Source: CAD feature listing. Evaluate the final solid. Frame: model axes, mm. Face numbers are marked on the shaded views. Give positions to 0.01 mm unless a question says otherwise; leave off trailing zeros. Loops run counter-clockwise (first coordinate to the right, second up) from the corner with the lowest first, then second, coordinate; pieces in that order, holes last.
from build123d import *

# Parameters (mm, degrees)
BOSS_EXTRUDE1_DEPTH = 10
BOSS_EXTRUDE2_START = -3
SKETCH2_R           = 3.5
SKETCH2_R_2         = 7.5
BOSS_EXTRUDE2_DEPTH = 3
BOSS_EXTRUDE5_START = -3
BOSS_EXTRUDE5_DEPTH = 10
SKETCH6_R           = 8.5
CUT_EXTRUDE1_DEPTH  = 246.440929757
SKETCH7_R           = 1
CUT_EXTRUDE2_DEPTH  = 246.544802429
BOSS_EXTRUDE6_DEPTH = 22
BOSS_EXTRUDE7_DEPTH = 2
FILLET1_R           = 2
FILLET3_R           = 2
SKETCH11_W          = 12
SKETCH11_H          = 7
CUT_EXTRUDE3_DEPTH  = 247.512170095
BOSS_EXTRUDE8_START = -10
BOSS_EXTRUDE8_DEPTH = 29.65
SKETCH13_R          = 2.5
CUT_EXTRUDE4_DEPTH  = 250.845097028
SKETCH14_W          = 120
SKETCH14_H          = 65
SKETCH14_R          = 5
BOSS_EXTRUDE9_DEPTH = 29.65
SKETCH15_W          = 60
SKETCH15_H          = 55
CUT_EXTRUDE5_DEPTH  = 19.65


with BuildPart() as part:
    # Sketch1 → Boss-Extrude1 (new body)
    with BuildSketch(Plane(origin=(0, 0, 0), x_dir=(1, 0, 0), z_dir=(0, 1, 0))):
        with BuildLine():
            Line((30, 26.5), (30, -243.5))
            Line((30, -243.5), (-30, -243.5))
            Line((-30, -243.5), (-30, 26.5))
            ThreePointArc((-30, 26.5), (0, 56.5), (30, 26.5))
        make_face()
        with BuildLine():
            ThreePointArc((11.477382224, -17.586065429), (21, 0), (11.477382224, 17.586065429))
            Line((11.477382224, 17.586065429), (5.68518373, 33.5))
            Line((5.68518373, 33.5), (-5.68518373, 33.5))
            Line((-5.68518373, 33.5), (-11.477382224, 17.586065429))
            ThreePointArc((-11.477382224, 17.586065429), (-21, 0), (-11.477382224, -17.586065429))
            Line((-11.477382224, -17.586065429), (-5.68518373, -33.5))
            Line((-5.68518373, -33.5), (5.68518373, -33.5))
            Line((5.68518373, -33.5), (11.477382224, -17.586065429))
        make_face(mode=Mode.SUBTRACT)
    extrude(amount=BOSS_EXTRUDE1_DEPTH)

    # Sketch2 → Boss-Extrude2 (add)
    with BuildSketch(Plane(origin=(0, 10, 0), x_dir=(1, 0, 0), z_dir=(0, 1, 0)).offset(BOSS_EXTRUDE2_START)):
        with BuildLine():
            Line((5.68518373, 33.5), (11.477382224, 17.586065429))
            ThreePointArc((11.477382224, 17.586065429), (21, 0), (11.477382224, -17.586065429))
            Line((11.477382224, -17.586065429), (5.68518373, -33.5))
            Line((5.68518373, -33.5), (-5.68518373, -33.5))
            Line((-5.68518373, -33.5), (-11.477382224, -17.586065429))
            ThreePointArc((-11.477382224, -17.586065429), (-21, 0), (-11.477382224, 17.586065429))
            Line((-11.477382224, 17.586065429), (-5.68518373, 33.5))
            Line((-5.68518373, 33.5), (5.68518373, 33.5))
        make_face()
        with Locations(Location((0, 26.5, 0), (0, 0, 270))):
            Circle(SKETCH2_R, mode=Mode.SUBTRACT)
        with Locations(Location((0, -26.5, 0), (0, 0, 90))):
            Circle(SKETCH2_R, mode=Mode.SUBTRACT)
        with Locations(Location((0, 0, 0), (0, 0, 270))):
            Circle(SKETCH2_R_2, mode=Mode.SUBTRACT)
    extrude(amount=BOSS_EXTRUDE2_DEPTH)

    # Sketch5 → Boss-Extrude5 (add)
    with BuildSketch(Plane.XZ.offset(-7).offset(BOSS_EXTRUDE5_START)):
        with BuildLine():
            Line((11.477382224, -17.586065429), (5.68518373, -33.5))
            Line((5.68518373, -33.5), (-5.68518373, -33.5))
            Line((-5.68518373, -33.5), (-11.477382224, -17.586065429))
            ThreePointArc((-11.477382224, -17.586065429), (0, -21), (11.477382224, -17.586065429))
        make_face()
        with BuildLine():
            Line((5.68518373, 33.5), (11.477382224, 17.586065429))
            ThreePointArc((11.477382224, 17.586065429), (0, 21), (-11.477382224, 17.586065429))
            Line((-11.477382224, 17.586065429), (-5.68518373, 33.5))
            Line((-5.68518373, 33.5), (5.68518373, 33.5))
        make_face()
    extrude(amount=BOSS_EXTRUDE5_DEPTH)

    # Sketch6 → Cut-Extrude1 (cut, through all)
    with BuildSketch(Plane.XZ.offset(-7)):
        with Locations(Location((0, 0, 0), (0, 0, 270))):
            Circle(SKETCH6_R)
    extrude(amount=-CUT_EXTRUDE1_DEPTH, mode=Mode.SUBTRACT)

    # Sketch7 → Cut-Extrude2 (cut, through all)
    with BuildSketch(Plane.XZ):
        with Locations(Location((0, 129.5, 0), (0, 0, 270))):
            Circle(SKETCH7_R)
        with Locations(Location((0, 177.5, 0), (0, 0, 90))):
            Circle(SKETCH7_R)
        with BuildLine():
            Line((-12.002194303, 178.230116364), (-24.730116364, 165.502194303))
            Line((-24.730116364, 165.502194303), (-19.780368896, 160.552446834))
            ThreePointArc((-19.780368896, 160.552446834), (14.849242405, 138.650757595), (-7.052446834, 173.280368896))
            Line((-7.052446834, 173.280368896), (-12.002194303, 178.230116364))
        make_face()
    extrude(amount=-CUT_EXTRUDE2_DEPTH, mode=Mode.SUBTRACT)

    # Sketch9 → Boss-Extrude6 (add)
    with BuildSketch(Plane.XZ):
        with BuildLine():
            Line((-21.664213552, 161.224108438), (-19.780368896, 160.552446834))
            ThreePointArc((-19.780368896, 160.552446834), (14.849242405, 138.650757595), (-7.052446834, 173.280368896))
            Line((-7.052446834, 173.280368896), (-7.724108438, 175.164213552))
            ThreePointArc((-7.724108438, 175.164213552), (16.263455967, 137.236544033), (-21.664213552, 161.224108438))
        make_face()
    extrude(amount=-BOSS_EXTRUDE6_DEPTH)

    # Sketch10 → Boss-Extrude7 (add)
    with BuildSketch(Plane(origin=(0, 22, 0), x_dir=(1, 0, 0), z_dir=(0, 1, 0))):
        with BuildLine():
            Line((-21.664213552, -161.224108438), (-16.012679582, -159.209123628))
            ThreePointArc((-16.012679582, -159.209123628), (12.02081528, -141.47918472), (-5.709123628, -169.512679582))
            Line((-5.709123628, -169.512679582), (-7.724108438, -175.164213552))
            ThreePointArc((-7.724108438, -175.164213552), (16.263455967, -137.236544033), (-21.664213552, -161.224108438))
        make_face()
    extrude(amount=BOSS_EXTRUDE7_DEPTH)

    # Fillet1
    fillet1_edges = [part.edges().sort_by_distance(p)[0] for p in [
        (16.263455967, 24, 137.236544033),
    ]]
    fillet(fillet1_edges, radius=FILLET1_R)

    # Fillet3
    # the kernel refuses this fillet: 2 mm, written as the material it adds along each edge
    with BuildSketch(Plane(origin=(0, 10, 153.5), x_dir=(-2.3359514129780358e-09, 0, 1.0), z_dir=(1.0, 0, 2.3359514129780358e-09))) as fillet3_piece_1_section:
        with BuildLine():
            CenterArc((23 + FILLET3_R, -FILLET3_R), FILLET3_R, 90, 90)
            Line((23 + FILLET3_R, 0), (23, 0))
            Line((23, 0), (23, -FILLET3_R))
        make_face()
    fillet3_piece_1 = revolve(axis=Axis((0, 10, 153.5), (0, -1, 0)), revolution_arc=19.623066341, mode=Mode.PRIVATE)
    fillet3_piece_1 = fillet3_piece_1 - Plane(origin=(0, 10.450783466, 177.5), x_dir=(0, 0, 1), z_dir=(0, -1, 0)) * Cylinder(1, 101, mode=Mode.PRIVATE)
    add(fillet3_piece_1)
    with BuildSketch(Plane(origin=(0, 10, 153.5), x_dir=(-0.9419223283656014, 0, 0.3358308016342816), z_dir=(0.3358308016342816, 0, 0.9419223283656014))) as fillet3_piece_2_section:
        with BuildLine():
            CenterArc((23 + FILLET3_R, -FILLET3_R), FILLET3_R, 90, 90)
            Line((23 + FILLET3_R, 0), (23, 0))
            Line((23, 0), (23, -FILLET3_R))
        make_face()
    fillet3_piece_2 = revolve(axis=Axis((0, 10, 153.5), (0, -1, 0)), revolution_arc=109.623066475, mode=Mode.PRIVATE)
    fillet3_piece_2 = fillet3_piece_2 - Plane(origin=(0, 10.562032205, 129.5), x_dir=(0, 0, -1), z_dir=(0, -1, 0)) * Cylinder(1, 101, mode=Mode.PRIVATE)
    add(fillet3_piece_2)
    with BuildSketch(Plane(origin=(0, 10, 153.5), x_dir=(0, 0, -1), z_dir=(-1, 0, 0))) as fillet3_piece_3_section:
        with BuildLine():
            CenterArc((23 + FILLET3_R, -FILLET3_R), FILLET3_R, 90, 90)
            Line((23 + FILLET3_R, 0), (23, 0))
            Line((23, 0), (23, -FILLET3_R))
        make_face()
    fillet3_piece_3 = revolve(axis=Axis((0, 10, 153.5), (0, -1, 0)), revolution_arc=180.000000134, mode=Mode.PRIVATE)
    fillet3_piece_3 = fillet3_piece_3 - Plane(origin=(0, 10.557784065, 177.5), x_dir=(0, 0, 1), z_dir=(0, -1, 0)) * Cylinder(1, 101, mode=Mode.PRIVATE)
    fillet3_piece_3 = fillet3_piece_3 - Plane(origin=(0, 10.557784065, 129.5), x_dir=(0, 0, -1), z_dir=(0, -1, 0)) * Cylinder(1, 101, mode=Mode.PRIVATE)
    add(fillet3_piece_3)

    # Sketch11 → Cut-Extrude3 (cut, through all)
    with BuildSketch(Plane.XZ):
        with Locations((0, 193.5)):
            Rectangle(SKETCH11_W, SKETCH11_H)
    extrude(amount=-CUT_EXTRUDE3_DEPTH, mode=Mode.SUBTRACT)

    # Sketch12 → Boss-Extrude8 (add)
    with BuildSketch(Plane.XZ.offset(BOSS_EXTRUDE8_START)):
        with BuildLine():
            Line((35, 243.5), (35, -26.5))
            ThreePointArc((35, -26.5), (0, -61.5), (-35, -26.5))
            Line((-35, -26.5), (-35, 243.5))
            Line((-35, 243.5), (-30, 243.5))
            Line((-30, 243.5), (-30, -26.5))
            ThreePointArc((-30, -26.5), (-29.473014303, -32.09834153), (-27.910571474, -37.5))
            Line((-27.910571474, -37.5), (27.910571474, -37.5))
            ThreePointArc((27.910571474, -37.5), (29.473014303, -32.09834153), (30, -26.5))
            Line((30, -26.5), (30, 243.5))
            Line((30, 243.5), (35, 243.5))
        make_face()
    extrude(amount=BOSS_EXTRUDE8_DEPTH)

    # Sketch13 → Cut-Extrude4 (cut, through all)
    with BuildSketch(Plane.XZ.offset(19.65)):
        with Locations(Location((-13.955285737, -42.559356041, 0), (0, 0, 270))):
            Circle(SKETCH13_R)
        with Locations(Location((13.955285737, -42.559356041, 0), (0, 0, 90))):
            Circle(SKETCH13_R)
    extrude(amount=-CUT_EXTRUDE4_DEPTH, mode=Mode.SUBTRACT)

    # Sketch14 → Boss-Extrude9 (add)
    with BuildSketch(Plane(origin=(0, 10, 0), x_dir=(1, 0, 0), z_dir=(0, 1, 0))):
        with Locations((0, -274)):
            Rectangle(SKETCH14_W, SKETCH14_H)
        with Locations(Location((46.25, -290.25, 0), (0, 0, 270))):
            Circle(SKETCH14_R, mode=Mode.SUBTRACT)
        with Locations(Location((-46.25, -290.25, 0), (0, 0, 90))):
            Circle(SKETCH14_R, mode=Mode.SUBTRACT)
        with Locations(Location((46.25, -257.75, 0), (0, 0, 90))):
            Circle(SKETCH14_R, mode=Mode.SUBTRACT)
        with Locations(Location((-46.25, -257.75, 0), (0, 0, 270))):
            Circle(SKETCH14_R, mode=Mode.SUBTRACT)
    extrude(amount=-BOSS_EXTRUDE9_DEPTH)

    # Sketch15 → Cut-Extrude5 (cut)
    with BuildSketch(Plane.XZ.offset(19.65)):
        with Locations((0, 269)):
            Rectangle(SKETCH15_W, SKETCH15_H)
    extrude(amount=-CUT_EXTRUDE5_DEPTH, mode=Mode.SUBTRACT)


solid = part.part
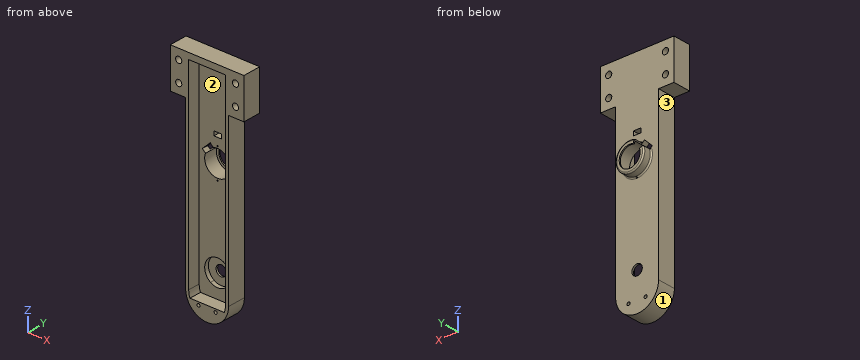
1) Cut plane A-A (x = -46.25). Return loops of the section in (y, z).
Checks:
outline: (-19.65, 241.5) - (10, 241.5) - (10, 252.75) - (-19.65, 252.75) - close; (-19.65, 262.75) - (10, 262.75) - (10, 285.25) - (-19.65, 285.25) - close; (-19.65, 295.25) - (10, 295.25) - (10, 306.5) - (-19.65, 306.5) - close
2) Contact query for flat-ended pins moving along their axis: P1, Ø6, axis at x = -13.96, z = -42.56, coming from the +Y side; P2, Ø6, axis at y = -13, z = 57, coming from the -X side; P3, Ø3, axis at x = 0, z = 129.5, coming from the +Y side; P4, Ø20.5, axis at x = 0, z = 153.5, coming from the +Y side. Output: stop coordinate, or through.
Checks:
P1: stops at y = 10
P2: stops at x = -35
P3: stops at y = 23.32
P4: passes through
3) Cut plane D-D (z = 121.5). Return loops of the section in (x, y), and give its area (4 significant figures).
Checks:
outline: (-35, -19.65) - (-30, -19.65) - (-30, 0) - (30, 0) - (30, -19.65) - (35, -19.65) - (35, 10) - (-35, 10) - close
area: 896.5 mm2
4) Cut plane C-C (y = -13). Return loops of the section in (x, z), and give its area (3 significant figures).
Checks:
outline: (-60, 241.5) - (-35, 241.5) - (-35, -26.5) arc R35 ccw to (35, -26.5) - (35, 241.5) - (60, 241.5) - (60, 306.5) - (-60, 306.5) - close; hole circle Ø10 at (-46.25, 257.75); hole circle Ø10 at (-46.25, 290.25); hole (-30, -26.5) arc R30 ccw to (-27.91, -37.5) - (27.91, -37.5) arc R30 ccw to (30, -26.5) - (30, 296.5) - (-30, 296.5) - close; hole circle Ø5 at (-13.96, -42.56); hole circle Ø5 at (13.96, -42.56); hole circle Ø10 at (46.25, 257.75); hole circle Ø10 at (46.25, 290.25)
area: 8,110 mm2
5) Cut plane B-B (z = 290.25). Return loops of the section in (x, y).
Checks:
outline: (-60, -19.65) - (-51.25, -19.65) - (-51.25, 10) - (-60, 10) - close; (-41.25, -19.65) - (-30, -19.65) - (-30, 0) - (30, 0) - (30, -19.65) - (41.25, -19.65) - (41.25, 10) - (-41.25, 10) - close; (51.25, -19.65) - (60, -19.65) - (60, 10) - (51.25, 10) - close
6) Pull-direction query (X, two-part tool) for the marked faces 1, 2 and 3; classes: released by +X, released by -X, zero draft, split by the parting line, or undercut.
Checks:
face 1: split by the parting line
face 2: undercut
face 3: released by -X
7) Ray query, probe 1 along Z at (x, y) = (0, 4); probe 2 along X at (y, z) = (6.5, 129.5); probe 3 along X at (y, z) = (-4, 290). Return the intervals inside material, ascending.
Checks:
probe 1: z = -61.5 to -21, 21 to 128.5, 130.5 to 132.5, 174.5 to 176.5, 178.5 to 190, 197 to 306.5
probe 2: x = -35 to -1, 1 to 35
probe 3: x = -60 to -51.24, -41.26 to -30, 30 to 41.26, 51.24 to 60
